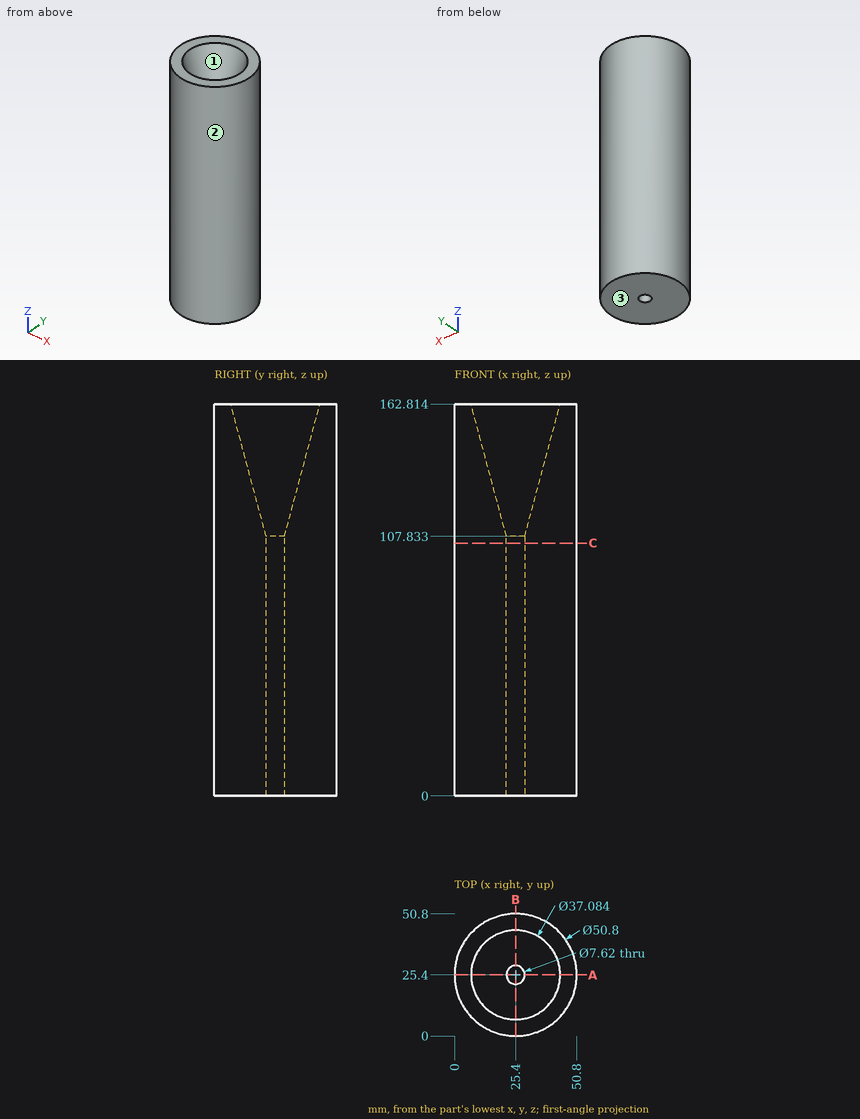
Verification items for this drawing (mm, ordinates from the low corner). Give positions to 0.01 mm unless a question says otherwise; leave off trailing zeros. Loops run counter-clockwise (first coordinate to the right, second up) from the corner with the lowest first, then second, coordinate; pieces in that order, holes last.
(1) Release check for a two-part mould opening along Y. For the marked faces 1, 2 and 3 record: released by +Y, released by -Y, zero draft, split by the parting line, or undercut.
From the geometry:
face 1: undercut
face 2: split by the parting line
face 3: zero draft
(2) Thickness scan on L1, parallel to Y at x = 25.4, z = 72; L2, parallel to Y at x = 26.5, z = 88 (1 decimal); L3, parallel to X at y = 32, z = 138 (1 decimal). Record the ranges inside material, lowest first.
From the geometry:
L1: y = 0 to 21.59, 29.21 to 50.8
L2: y = 0 to 21.8, 29 to 50.8
L3: x = 0.9 to 15.5, 35.3 to 49.9
(3) Depth check by flat-ended pin: pin 1 Ø3 at (y, z) = (45.5, 74.5) entering from -X; pin 2 Ø2 at (y, z) = (35.5, 40.5) entering from +X; pin 3 Ø1.5 at (y, z) = (27.5, 141) entering from +X. Enter the tip coordinate at first touch or a pass-through.
From the geometry:
pin 1: stops at x = 8.1
pin 2: stops at x = 49.11
pin 3: stops at x = 50.76
(4) Section check A-A on y = 25.4. Record the cut outline in (x, z).
From the geometry:
outline: (0, 0) - (21.59, 0) - (21.59, 107.83) - (6.86, 162.81) - (0, 162.81) - close; (29.21, 0) - (50.8, 0) - (50.8, 162.81) - (43.94, 162.81) - (29.21, 107.83) - close
(5) Section check C-C on z = 105. Record the cut outline in (x, y).
From the geometry:
outline: circle Ø50.8 at (25.4, 25.4); hole circle Ø7.62 at (25.4, 25.4)
